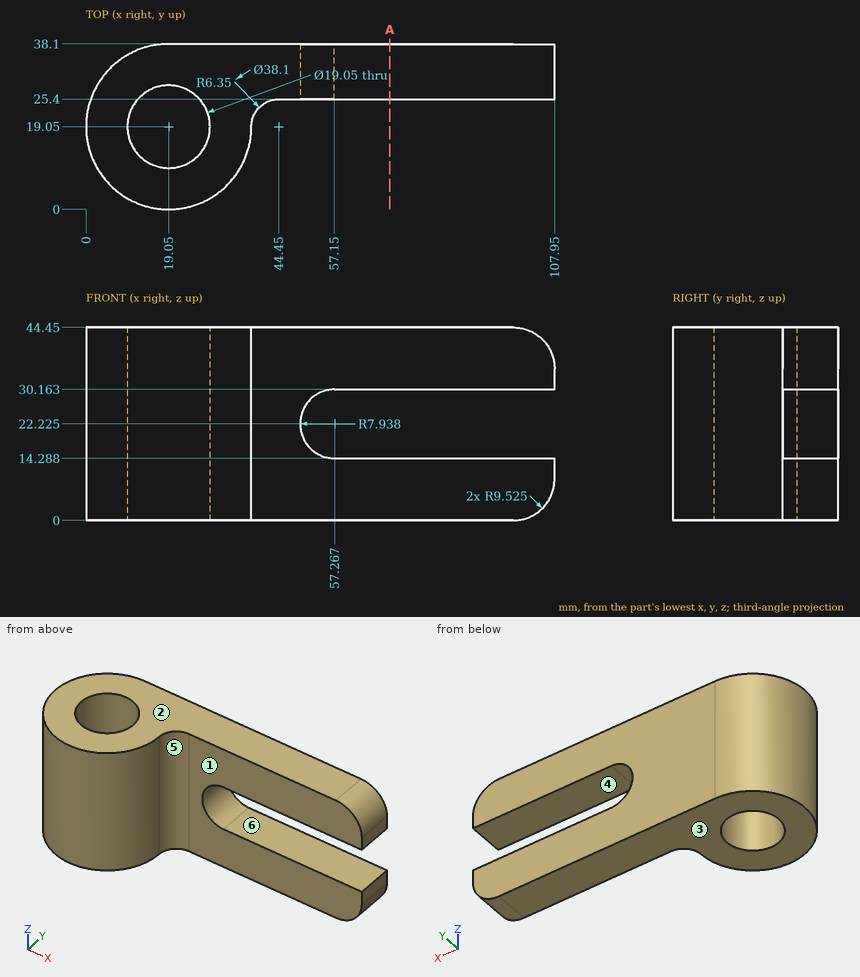
Input: dimensioned drawing with shaded views. Units: mm. Origin: part minimum x, y, z. A direction names the side the tool comes from. Coordinates: 2 decimals unless noted, no trailing zeros. Loops run counter-clockwise (first coordinate to the right, second up) from the corner with the lowest first, then second, coordinate; pieces in that order, holes last. Notation, with made-up numbers: M 60,-39 L 94,-39 A25 ccw 94,-6 Z; hole C 32.5,53.5 d3. An arc over 180 degrees is marked long. Use a Markdown table: item, result. Add a question column.
1) Draft query along Z for the marked faces 1, 2, 3 and 4. Return one class per face: +Z half, -Z half, draft (parallel to the pull), parting line (faces both ways), or undercut.
2) Set-up query: the marked faces 5 and 6. Return all of +Z, -Z, +X, -X, +Y, -Y with unobstructed straight access to the full face (end or side cutting, diameter ignored); none if empty.
3) Pin query (flat end, axial travel): P1, Ø8, axis at x = 29, z = 38.5, coming from the -Y side; P2, Ø5, axis at y = 30, z = 23, coming from the +X side; P3, Ø2, axis at x = 61.5, z = 12, coming from the -Y side. Return the tip coordinate at first contact, or that it passes through.
4) Line query: L1, parallel to Y at x = 19.05, z = 33 (1 decimal); L2, parallel to Y at x = 62, z = 38.5. Output: solid intervals per line, ascending. Write a range as from..to.
5) Section A-A, the plane x = 70. Return the cut outline in (y, z).
Answer below:
| question | item | result |
|---|---|---|
| 1 | face 1 | draft |
| 1 | face 2 | +Z half |
| 1 | face 3 | -Z half |
| 1 | face 4 | undercut |
| 2 | face 5 | +Z, -Z, +X, -Y |
| 2 | face 6 | +X, +Y, -Y |
| 3 | P1 | y = 0.95 |
| 3 | P2 | x = 50.04 |
| 3 | P3 | y = 25.4 |
| 4 | L1 | 0..9.5, 28.6..38.1 |
| 4 | L2 | 25.4..38.1 |
| 5 | outline | M 25.4,0 L 38.1,0 L 38.1,14.29 L 25.4,14.29 Z; M 25.4,30.16 L 38.1,30.16 L 38.1,44.45 L 25.4,44.45 Z |
